Verification items for the finished model (mm, model axes). A direction names the side the tool comes from. Round coordinates to 2 decimals unless told otherwise and drop trailing zeros. Loops run counter-clockwise (first coordinate to the right, second up) from the corner with the lowest first, then second, coordinate; pieces in that order, holes last. Notation, with made-up numbers: (56, -30) -> (94, -30) arc R26 cw to (94, -9) -> close; hole circle Ø8 at (0.5, 22). An arc over 180 degrees is marked (long way). Write item = value, one per line.
Autodesk Inventor part; units mm, degrees
ref_plane "YZ Plane" through (0, 0, 0) normal (1, 0, 0) x (0, 1, 0)
ref_plane "XZ Plane" through (0, 0, 0) normal (0, 1, 0) x (-1, 0, 0)
ref_plane "XY Plane" through (0, 0, 0) normal (0, 0, 1) x (1, 0, 0)
sketch "Sketch1" plane through (0, 0, 0) normal (0, 0, 1) x (1, 0, 0)
  line L0 (26.7421, 25.9605) -> (26.7421, 49.1206)
  line L1 (40.2452, 62.9605) -> (96.239, 62.9605)
  line L2 (39.9339, 67.9605) -> (96.5503, 67.9605)
  line L3 (106.7421, 25.9605) -> (106.7421, 47.9605)
  line L4 (26.7421, 25.9605) -> (29.7421, 25.9605)
  line L5 (106.7421, 25.9605) -> (109.7421, 25.9605)
  line L6 (109.7421, 25.9605) -> (109.7421, 49.1206)
  line L7 (29.7421, 25.9605) -> (29.7421, 47.9605)
  line L8 (29.7421, 47.9605) -> (40.2452, 62.9605)
  line L9 (26.7421, 49.1206) -> (39.9339, 67.9605)
  line L10 (106.7421, 47.9605) -> (96.239, 62.9605)
  line L11 (109.7421, 49.1206) -> (96.5503, 67.9605)
  point P0 (0, 0)
extrude "Extrusion1" add sketch "Sketch1" along normal blind 45
sketch "Sketch2" plane through (109.7421, 25.9605, 0) normal (1, 0, 0) x (0, 0, -1)
  line L0 (-45, 23.1601) -> (-45, 0)
  line L1 (0, 0) -> (-45, 0)
  line L2 (0, 23.1601) -> (0, 0)
  line L3 (0, 23.1601) -> (-45, 23.1601)
  line L4 (-45, 23.1601) -> (-31.3837, 4.513)
  line L5 (0, 23.1601) -> (-13.6163, 4.513)
  arc A0 (-18, 11) -> (-27, 11) centre (-22.5, 11) ccw
  line L6 (-45, 23.1601) -> (-45, -1.8399)
  line L7 (-45, -1.8399) -> (0, -1.8399)
  line L8 (0, -1.8399) -> (0, 23.1601)
  line L9 (-18, 11) -> (-18, 0.9626)
  line L10 (-27, 11) -> (-27, 0.9626)
  arc A1 (-18, 0.9626) -> (-13.6163, 4.513) centre (-22.5, 11) ccw
  arc A2 (-31.3837, 4.513) -> (-27, 0.9626) centre (-22.5, 11) ccw
  line L11 (-45, 42) -> (-33.5, 42)
  line L12 (-33.5, 42) -> (-33.5, 2)
  line L13 (-33.5, 2) -> (-45, 2)
  line L14 (-45, 2) -> (-45, 42)
  line L15 (0, 42) -> (-11.5, 42)
  line L16 (-11.5, 42) -> (-11.5, 2)
  line L17 (-11.5, 2) -> (0, 2)
  line L18 (0, 2) -> (0, 42)
  circle A3 centre (-22.5, 11) radius 11
  point P0 (0, -25.9605)
  dimension "d3" = 11
  dimension "d4" = 9
  dimension "d5" = 25
  dimension "d14" = 11.5
  dimension "d15" = 11.5
  dimension "d16" = 40
  dimension "d17" = 40
sketch "Sketch3" plane through (39.9339, 67.9605, 0) normal (0, 1, 0) x (1, 0, 0)
  circle A0 centre (46.0082, -22.5) radius 5
  line L0 (69.8082, 0) -> (69.8082, -45)
  point P0 (-39.9339, 0)
  dimension "d8" = 10
  dimension "d9" = 23.8
extrude "Extrusion3" cut sketch "Sketch3" against normal blind 45
extrude "Extrusion4" cut sketch "Sketch2" against normal through all contours L4 L12 L13 L0 | L14 L11 L12 L3 | L3 L12 L4 | L13 L12 L4 A2 A3 L1 L0 | L16 L15 L18 L3 | L3 L5 L16 | A3 A1 L5 L16 L17 L2 L1 | A3 L10 A0 L9 | L2 L17 L16 L5
sketch "Sketch4" plane through (109.7421, 33.3718, 33.5) normal (1, 0, 0) x (0, 0, -1)
  arc A0 (15.5, -6.4487) -> (19.8837, -2.8983) centre (11, 3.5887) ccw
  line L0 (11, 3.5887) -> (19.5, 3.5887) construction
  circle A1 centre (7.7472, 11.4417) radius 1
  point P0 (33.5, -33.3718)
  dimension "d22" = 2
extrude "Extrusion5" cut sketch "Sketch4" against normal through all
pattern_circular "Circular Pattern1" count 8 over 360 about axis through (109.7421, 36.9605, 22.5) along (-1, 0, 0) of "Extrusion5"
sketch "Sketch5" plane through (40.2452, 62.9605, 11.5) normal (0, -1, 0) x (1, 0, 0)
  circle A0 centre (45.6969, 11) radius 5
  circle A1 centre (37.1969, 11) radius 1
  point P0 (-40.2452, -11.5)
  dimension "d28" = 2
  dimension "d29" = 8.5
extrude "Extrusion6" cut sketch "Sketch5" against normal through all contours A1
pattern_circular "Circular Pattern2" count 8 over 360 about axis through (85.9421, 67.9605, 22.5) along (0, -1, 0) of "Extrusion6"
properties part number "Hips" material "Aluminum-6061"
(1) Go/stop test with flat-tipped pins: pin 1 Ø4 at (x, z) = (100, 31) entering from +Y; pin 2 Ø8 at (x, z) = (36.5, 21) entering from +Y; pin 3 Ø1.8 at (x, z) = (85.94, 14) entering from -Y; pin 4 Ø1.5 at (x, y) = (29, 30) entering from -Z. Record where each tip stops, or that it passes through.
Filled sheet:
pin_1 = 65.89
pin_2 = 67.96
pin_3 = through
pin_4 = 13.41
(2) Sectioned sample at D-D, the plane y = 57. Record the cut outline in (x, z).
Filled sheet:
outline = (32.26, 11.5) -> (36.07, 11.5) -> (36.07, 33.5) -> (32.26, 33.5) -> close; (100.41, 11.5) -> (104.22, 11.5) -> (104.22, 33.5) -> (100.41, 33.5) -> close
(3) Draft check along Y on faces 1 (the face through (108.263, 45.551, 19.922)), 2 (the face through (101.56, 55.36, 22.35)), 3 (the face through (86.934, 65.426, 31.13)). Enter one of: released by +Y, released by -Y, zero draft, split by the parting line, or undercut.
Filled sheet:
face_1 = undercut
face_2 = released by -Y
face_3 = zero draft
(4) Material ranges on probe 1 along X at (y, z) = (42, 17.5); probe 2 along Y at (x, z) = (44.5, 30); probe 3 along X at (y, z) = (56.5, 31.25) (3 decimals), recorded low to high. Write a range as from..to.
Filled sheet:
probe_1 = 26.74..29.74, 106.74..109.74
probe_2 = 62.96..67.96
probe_3 = 31.909..35.722, 100.763..104.575
(5) Sectioned sample at A-A, the plane y = 36. Record the cut outline in (x, z), and give its area (3 significant figures).
Filled sheet:
outline = (26.74, 11.5) -> (29.74, 11.5) -> (29.74, 18) -> (26.74, 18) -> close; (26.74, 27) -> (29.74, 27) -> (29.74, 33.5) -> (26.74, 33.5) -> close; (106.74, 11.5) -> (109.74, 11.5) -> (109.74, 18) -> (106.74, 18) -> close; (106.74, 27) -> (109.74, 27) -> (109.74, 33.5) -> (106.74, 33.5) -> close
area = 78.0 mm2
(6) Set-up check for faces 4 (the face through (28, 32, 27)), 5 (the face through (28.263, 40.43, 15.623)): record each of +Z, -Z, +X, -X, +Y, -Y from which the full face is reachable in a straight line by a thin tool's end or side.
Filled sheet:
face_4 = +X, -X, -Y
face_5 = +X, -X
(7) Sectioned sample at C-C, the plane x = 77.5. Record the cut outline in (y, z).
Filled sheet:
outline = (62.96, 11.5) -> (67.96, 11.5) -> (67.96, 21.5) -> (62.96, 21.5) -> close; (62.96, 23.5) -> (67.96, 23.5) -> (67.96, 33.5) -> (62.96, 33.5) -> close
(8) Sectioned sample at B-B, the plane z = 22.5. Record the cut outline in (x, y), and give its area (3 significant figures).
Filled sheet:
outline = (26.74, 41.46) -> (29.74, 41.46) -> (29.74, 47.96) -> (40.25, 62.96) -> (76.44, 62.96) -> (76.44, 67.96) -> (39.93, 67.96) -> (26.74, 49.12) -> close; (78.44, 62.96) -> (80.94, 62.96) -> (80.94, 67.96) -> (78.44, 67.96) -> close; (90.94, 62.96) -> (93.44, 62.96) -> (93.44, 67.96) -> (90.94, 67.96) -> close; (95.44, 62.96) -> (96.24, 62.96) -> (106.74, 47.96) -> (106.74, 41.46) -> (109.74, 41.46) -> (109.74, 49.12) -> (96.55, 67.96) -> (95.44, 67.96) -> close
area = 383 mm2
